Geometry check sheet. Reference: the model listing, model coordinates, mm. A direction names the side the tool comes from. Coordinates: 2 decimals unless noted, no trailing zeros. Loops run counter-clockwise (first coordinate to the right, second up) from the corner with the lowest first, then second, coordinate; pieces in that order, holes last.
from build123d import *

# Parameters (mm, degrees)
F0_W     = 10.16
F0_H     = 20.32
F0_W_2   = 20.32
F0_H_2   = 10.16
F1_DEPTH = 6.35
F2_R     = 15.875
F3_DEPTH = 6.35
F4_R     = 11.1125
F5_DEPTH = 6.351
F6_R     = 10.16
F7_DEPTH = 6.35
F8_R     = 5.08
F9_DEPTH = 6.351


with BuildPart() as f1:
    # F0 (on Front) → F1 (new body)
    with BuildSketch(Plane.XZ):
        with Locations((20.32, -15.24)):
            Rectangle(F0_W, F0_H)
        Polygon((15.24, -5.08), (25.4, -5.08), (25.4, 5.08), (5.08, 5.08), (5.08, -5.08), align=None)
        Polygon((5.08, -25.4), (5.08, -5.08), (-5.08, -5.08), (-5.08, -15.24), (-5.08, -25.4), align=None)
        Polygon((-5.08, 5.08), (5.08, 5.08), (5.08, 15.24), (5.08, 25.4), (-5.08, 25.4), align=None)
        Polygon((-25.4, -5.08), (-5.08, -5.08), (-5.08, 5.08), (-15.24, 5.08), (-25.4, 5.08), align=None)
        with Locations((15.24, 20.32)):
            Rectangle(F0_W_2, F0_H_2)
        with Locations((-15.24, -20.32)):
            Rectangle(F0_W_2, F0_H_2)
        with Locations((-20.32, 15.24)):
            Rectangle(F0_W, F0_H)
    extrude(amount=F1_DEPTH)

    # F2 (on Front) → F3 (join)
    with BuildSketch(Plane.XZ):
        with Locations((-25.4, 25.4)):
            Circle(F2_R)
        with BuildLine():
            ThreePointArc((41.275, 25.4), (25.4, 41.275), (9.525, 25.4))
            ThreePointArc((9.525, 25.4), (25.4, 9.525), (41.275, 25.4))
        make_face()
        with BuildLine():
            ThreePointArc((41.275, -25.4), (25.4, -9.525), (9.525, -25.4))
            ThreePointArc((9.525, -25.4), (25.4, -41.275), (41.275, -25.4))
        make_face()
        with Locations((-25.4, -25.4)):
            Circle(F2_R)
    extrude(amount=F3_DEPTH)

    # F4 (on Front) → F5 (cut, through all)
    with BuildSketch(Plane.XZ):
        with Locations((-25.4, 25.4)):
            Circle(F4_R)
        with BuildLine():
            ThreePointArc((36.5125, 25.4), (25.4, 36.5125), (14.2875, 25.4))
            ThreePointArc((14.2875, 25.4), (25.4, 14.2875), (36.5125, 25.4))
        make_face()
        with BuildLine():
            ThreePointArc((36.5125, -25.4), (25.4, -14.2875), (14.2875, -25.4))
            ThreePointArc((14.2875, -25.4), (25.4, -36.5125), (36.5125, -25.4))
        make_face()
        with Locations((-25.4, -25.4)):
            Circle(F4_R)
    extrude(amount=F5_DEPTH, mode=Mode.SUBTRACT)

    # F6 (on Front) → F7 (join)
    with BuildSketch(Plane.XZ):
        Circle(F6_R)
    extrude(amount=F7_DEPTH)

    # F8 (on Front) → F9 (cut, through all)
    with BuildSketch(Plane.XZ):
        Circle(F8_R)
    extrude(amount=F9_DEPTH, mode=Mode.SUBTRACT)


solid = f1.part
(1) Scan lines: L1, parallel to Z at x = 26, y = -2.5; L2, parallel to Z at x = 17, y = -0.5; L3, parallel to X at y = -5.5, z = 16. Record each from-to range of solid material in increasing order.
Findings:
L1: z = -41.26 to -36.5, -14.3 to -9.54, 9.54 to 14.3, 36.5 to 41.26
L2: z = -38.87 to -32.68, -18.12 to 5.08, 11.93 to 18.12, 32.68 to 38.87
L3: x = -38.19 to -31.33, -19.47 to -12.61, -5.08 to 19.47, 31.33 to 38.19
(2) Access from +Z, -Z, +X, -X, +Y, -Y to the whole of each face (thin tool, end or side, straight path). Record for faces 3 (the cylindrical face through (-7.21, -3.13, -7.16)), 4 (the flat face through (5.08, -3, -17)), 5 (the flat face through (-5.08, -3, 17)), 6 (the flat face through (-5.08, -3, -12)).
Findings:
face 3: -X, +Y, -Y
face 4: -Z, +Y, -Y
face 5: +Z, +Y, -Y
face 6: +Y, -Y
(3) Sectioned sample at D-D on y = -3.75. State how many separate pieces and enclosed holes the cut face has, and give its area (3 significant figures).
Findings:
separate pieces: 1
enclosed holes: 5
area: 2,720 mm2
(4) Draft check along Z on faces 1 (the flat face through (0, -6.35, -6)), 2 (the flat face through (5.08, -3, 12)). Enter one of: +Z half, -Z half, draft (parallel to the pull), parting line (faces both ways), or undercut.
Findings:
face 1: draft
face 2: undercut
(5) Sectioned sample at A-A on z = 0. Record the cut outline in (x, y).
Findings:
outline: (-25.4, -6.35) - (-5.08, -6.35) - (-5.08, 0) - (-25.4, 0) - close; (5.08, -6.35) - (25.4, -6.35) - (25.4, 0) - (5.08, 0) - close
(6) Gauge pin test, flat ends, axial feed: pin 1 Ø1 at (y, z) = (-3.5, -3) entering from +X; pin 2 Ø1.9 at (x, y) = (-15.5, -2) entering from -Z; pin 3 Ø3 at (y, z) = (-2, 13.5) entering from -X. Record the tip position at first contact, or that the pin passes through.
Findings:
pin 1: stops at x = 25.4
pin 2: stops at z = -38.51
pin 3: stops at x = -37.39
(7) Sectioned sample at C-C on x = 0. Record the cut outline in (y, z).
Findings:
outline: (-6.35, -25.4) - (0, -25.4) - (0, -5.08) - (-6.35, -5.08) - close; (-6.35, 5.08) - (0, 5.08) - (0, 25.4) - (-6.35, 25.4) - close
(8) Sectioned sample at B-B on x = 32.5. Record the cut outline in (y, z), and give its area (3 significant figures).
Findings:
outline: (-6.35, -39.6) - (0, -39.6) - (0, -33.95) - (-6.35, -33.95) - close; (-6.35, -16.85) - (0, -16.85) - (0, -11.2) - (-6.35, -11.2) - close; (-6.35, 11.2) - (0, 11.2) - (0, 16.85) - (-6.35, 16.85) - close; (-6.35, 33.95) - (0, 33.95) - (0, 39.6) - (-6.35, 39.6) - close
area: 144 mm2
